Check sheet for the drawn part. Datum: minimum x, y, z corner. Units: mm. Coordinates: 2 decimals unless noted, no trailing zeros. Loops run counter-clockwise (first coordinate to the right, second up) from the corner with the lowest first, then second, coordinate; pieces in that order, holes last.
Q1. Sectioned sample at C-C (z = 1.2). Count the separate pieces of the cut face and the enclosed holes in it, then the cut area to 3 significant figures.
Q2. Material ranges on probe 1 along X at (y, z) = (51, 1.95); probe 2 along X at (y, z) = (52, 0.8) (1 decimal); probe 3 along X at (y, z) = (27.5, 0.45), recorded low to high.
Q3. Sectioned sample at D-D (x = 82.55). Enter the section's corners in (y, z) (1 decimal).
Q4. Sectioned sample at B-B (y = 50.8). Enter the section's corners in (x, z) (1 decimal).
Q5. Sectioned sample at A-A (x = 50.8). Enter the section's corners in (y, z) (1 decimal).
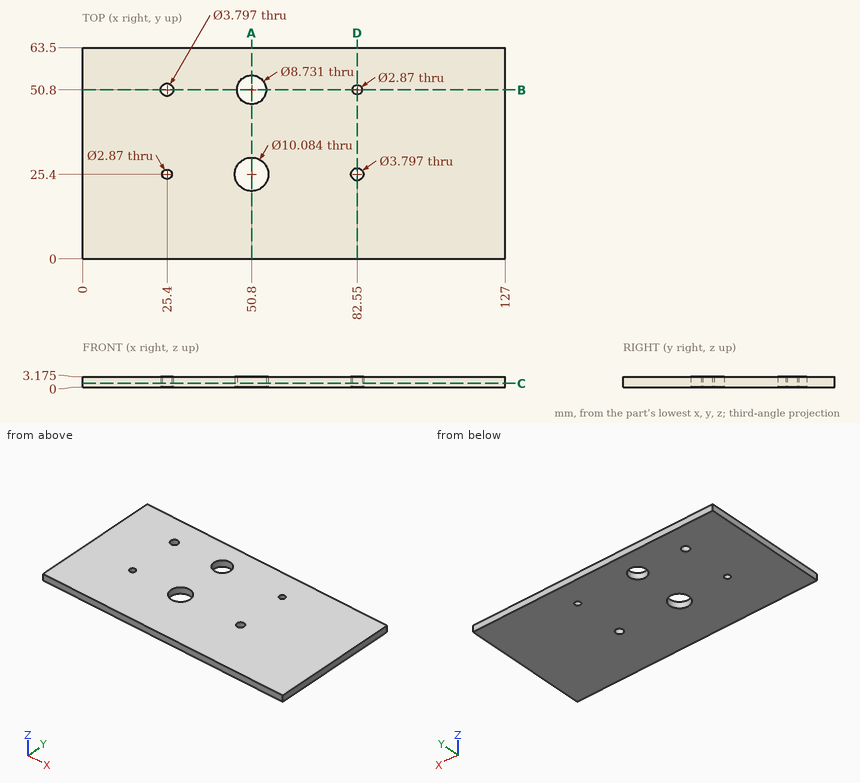
Geometry check:
1. separate pieces: 1
1. enclosed holes: 6
1. area: 7,890 mm2
2. probe 1: x = 0 to 23.51, 27.29 to 46.44, 55.16 to 81.13, 83.97 to 127
2. probe 2: x = 0 to 23.9, 26.9 to 46.6, 55 to 81.8, 83.3 to 127
2. probe 3: x = 0 to 46.22, 55.38 to 127
3. outline: (0, 0) - (23.5, 0) - (23.5, 3.2) - (0, 3.2) - close; (27.3, 0) - (49.4, 0) - (49.4, 3.2) - (27.3, 3.2) - close; (52.2, 0) - (63.5, 0) - (63.5, 3.2) - (52.2, 3.2) - close
4. outline: (0, 0) - (23.5, 0) - (23.5, 3.2) - (0, 3.2) - close; (27.3, 0) - (46.4, 0) - (46.4, 3.2) - (27.3, 3.2) - close; (55.2, 0) - (81.1, 0) - (81.1, 3.2) - (55.2, 3.2) - close; (84, 0) - (127, 0) - (127, 3.2) - (84, 3.2) - close
5. outline: (0, 0) - (20.4, 0) - (20.4, 3.2) - (0, 3.2) - close; (30.4, 0) - (46.4, 0) - (46.4, 3.2) - (30.4, 3.2) - close; (55.2, 0) - (63.5, 0) - (63.5, 3.2) - (55.2, 3.2) - close
